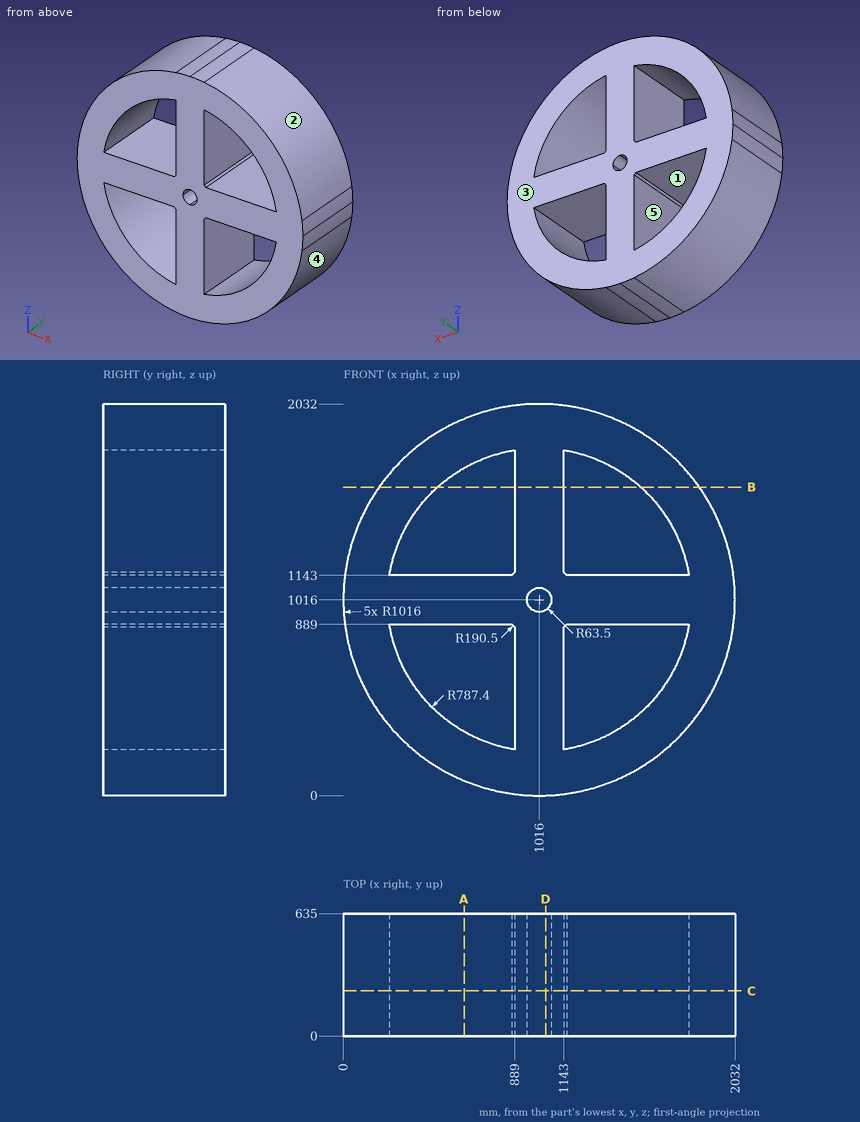
Input: dimensioned drawing with shaded views. Units: mm. Origin: part minimum x, y, z. A direction names the side the tool comes from. Coordinates: 2 decimals unless noted, no trailing zeros. Order: outer loops, then holes, each group sorted by start corner. A loop starts at its lowest first (then second) coordinate and runs counter-clockwise, first axis right, second up. Notation, with made-up numbers: M 87.5,-30.75 L 124.5,-30.75 A24 cw 124.5,-15.75 Z; hole C 66,-10 d10. An arc over 180 degrees is marked long. Write each question's results on one line, items separated by ' | '. Start each with the question number.
Item 1: Cut plane A-A (x = 627). Return loops of the section in (y, z).
Item 2: Line query: probe 1 along Z at (x, y) = (1481.5, 605) (1 decimal); probe 2 along Z at (x, y) = (1287.5, 572); probe 3 along X at (y, z) = (378.5, 325) (1 decimal). Output: solid intervals per line, ascending.
Item 3: First-contact query: pin 1 Ø10 at (y, z) = (248.5, 1374) entering from +X (1 decimal); pin 2 Ø5 at (y, z) = (382, 426.5) entering from +X; pin 3 Ø8 at (x, y) = (1250.5, 140.5) entering from -Z. Flat tips, straight axial feed; report the tip coordinate or a pass-through.
Item 4: Cut plane C-C (y = 234.5). Count the separate pieces of the cut face and the enclosed holes in it, and give its area (3 significant figures).
Item 5: Draft query along Z for the marked faces 3, 4 and 5. Return one class per face: pulls with the +Z half, pulls with the -Z half, needs draft (parallel to the pull), parting line crosses it, or undercut.
Item 6: Set-up query: the marked faces 1 and 2. Return all of +Z, -Z, +X, -X, +Y, -Y with unobstructed straight access to the full face (end or side cutting, diameter ignored); none if empty.
Item 7: Cut plane B-B (z = 1601). Return loops of the section in (x, y), and give its area (3 significant figures).
Item 8: Cut plane D-D (x = 1049). Return loops of the section in (y, z), and give its area (3 significant figures).
Checked values:
1) outline: M 0,77.42 L 635,77.42 L 635,331.4 L 0,331.4 Z; M 0,889 L 635,889 L 635,1143 L 0,1143 Z; M 0,1700.6 L 635,1700.6 L 635,1954.58 L 0,1954.58 Z
2) probe 1: z = 112.9 to 380.9, 889 to 1143, 1651.1 to 1919.1 | probe 2: z = 36.95 to 276.89, 889 to 1143, 1755.11 to 1995.05 | probe 3: x = 271.2 to 638.5, 889 to 1143, 1393.5 to 1760.8
3) pin 1: stops at x = 1968.7 | pin 2: stops at x = 1845.27 | pin 3: stops at z = 26.49
4) separate pieces: 1 | enclosed holes: 5 | area: 2,010,000 mm2
5) face 3: needs draft | face 4: pulls with the -Z half | face 5: undercut
6) face 1: +Y, -Y | face 2: +Z, +X, +Y, -Y
7) outline: M 185.32,0 L 488.96,0 L 488.96,635 L 185.32,635 Z; M 889,0 L 1143,0 L 1143,635 L 889,635 Z; M 1543.04,0 L 1846.68,0 L 1846.68,635 L 1543.04,635 Z | area: 547,000 mm2
8) outline: M 0,0.54 L 635,0.54 L 635,961.75 L 0,961.75 Z; M 0,1070.25 L 635,1070.25 L 635,2031.46 L 0,2031.46 Z | area: 1,220,000 mm2
